Check sheet for the modelled part. Datum: model origin and axes. Units: mm. A direction names the side the tool comes from. Round coordinates to 2 decimals unless told otherwise and drop trailing zeros. Loops run counter-clockwise (first coordinate to the right, second up) from the corner with the lowest first, then second, coordinate; pieces in that order, holes last. Notation, with made-up numbers: (9.5, 48.5) - (24.5, 48.5) arc R27 cw to (24.5, 64.5) - close; hole circle Ø10 at (58.5, -6.5). An arc over 180 degrees is marked (long way). Answer in a Markdown table with one row per item. Add a question column.
(1) Thickness scan on line 1 along Y through (x, z) = (1.75, 3.5); line 2 along Z through (x, y) = (5.5, -12); line 3 along Y through (x, z) = (5.25, -3). Record the ranges inside material, lowest first.
(2) Cross-section at C-C on y = -16.5. Enter the section's corners in (x, z), then the cut area to 3 significant figures.
(3) Mould release check, pull along Z, two halves, no side actions. Record for faces 1 (the flat face through (-4.02, 0, 4)), 2 (the flat face through (0.532, -2.776, 3.095)), 3 (the flat face through (5.259, -26.016, -31.007)): +Z half, -Z half, draft (parallel to the pull), parting line (faces both ways), or undercut.
(4) Gauge pin test, flat ends, axial feed: pin 1 (1.6 mm diameter, centred on x = 5.5, z = 4.5, fed in from +Y); pin 2 (0.6 mm diameter, centred on y = -3.5, z = 4, fed in from +X); pin 3 (1.5 mm diameter, centred on y = -24.5, z = -32, fed in from +X). Record the tip position at first contact, or that the pin passes through.
(5) Cross-section at B-B on z = -11. Enter the section's corners in (x, y).
(6) Access from +Z, -Z, +X, -X, +Y, -Y to the whole of each face (thin tool, end or side, straight path). Record for faces 4 (the cylindrical face through (-0.69, -25.64, -30.54)), 5 (the flat face through (0.5, -20.6, -33.8)), 6 (the flat face through (-0.08, -22.91, -26.23)), 7 (the flat face through (0, 0, 0)).
from build123d import *

# Parameters (mm, degrees)
SKETCH1_W                      = 12.04
SKETCH1_H                      = 7.58
SKETCH1_W_2                    = 8.04
SKETCH1_H_2                    = 3.58
BOSS_EXTRUDE1_DEPTH            = 8
SKETCH1_2_W                    = 12.04
SKETCH1_2_H                    = 7.58
SKETCH1_2_W_2                  = 8.04
SKETCH1_2_H_2                  = 3.58
BOSS_EXTRUDE2_DEPTH            = 2
EXTRUDE_THIN1_DEPTH            = 12.04
SKETCH5_W                      = 12.04
SKETCH5_H                      = 7.58
SKETCH5_W_2                    = 8.04
SKETCH5_H_2                    = 3.58
BOSS_EXTRUDE4_DEPTH            = 8
SKETCH5_4_W                    = 12.04
SKETCH5_4_H                    = 7.58
BOSS_EXTRUDE5_DEPTH            = 2
CHAMFER1_SIZE                  = 1.5
CHAMFER2_START                 = -7
CHAMFER2_DEPTH                 = 14
CUT_EXTRUDE1_REACH             = 50.973
CUT_EXTRUDE1_DIRECTION_2_DEPTH = 49.973440368
CUT_EXTRUDE2_DEPTH             = 48.541116576
CUT_EXTRUDE2_DEPTH_BACK        = 48.541116576
SKETCH8_W                      = 2
SKETCH8_H                      = 1.58
CUT_EXTRUDE3_DEPTH             = 6.5
SKETCH9_W                      = 4
SKETCH9_H                      = 1.58
CUT_EXTRUDE4_DEPTH             = 6.5
CHAMFER3_SIZE                  = 0.5
SKETCH10_W                     = 0.414634146
SKETCH10_H                     = 2
SKETCH10_W_2                   = 0.414634147
BOSS_EXTRUDE6_DEPTH            = 0.3


with BuildPart() as part:
    # Sketch1 → Boss-Extrude1 (new body)
    with BuildSketch(Plane.XY):
        Rectangle(SKETCH1_W, SKETCH1_H)
        Rectangle(SKETCH1_W_2, SKETCH1_H_2, mode=Mode.SUBTRACT)
    extrude(amount=BOSS_EXTRUDE1_DEPTH)

    # Sketch1<2> → Boss-Extrude2 (add)
    # profile 1 of 2: a face of its own
    with BuildSketch(Plane.XY):
        Rectangle(SKETCH1_2_W, SKETCH1_2_H)
        Rectangle(SKETCH1_2_W_2, SKETCH1_2_H_2, mode=Mode.SUBTRACT)
    # profile 2 of 2: a face of its own
    with BuildSketch(Plane.XY):
        Rectangle(SKETCH1_2_W_2, SKETCH1_2_H_2)
    extrude(amount=-BOSS_EXTRUDE2_DEPTH)

    # Sketch3 → Extrude-Thin1 (add)
    with BuildSketch(Plane(origin=(6.02, 9.81, 0), x_dir=(0, -1, 0), z_dir=(1, 0, 0))):
        with BuildLine():
            Line((6.02, 2.744137986), (6.52, 2.744137986))
            ThreePointArc((6.52, 2.744137986), (10.07949931, 2.557592532), (13.6, 2))
            Line((13.6, 2), (21.425180806, 0.336706473))
            ThreePointArc((21.425180806, 0.336706473), (22.120268588, 0.441550315), (22.574623539, 0.977927827))
            ThreePointArc((22.574623539, 0.977927827), (26.849152106, 14.317688881), (30.219561316, 27.914054616))
            Line((30.219561316, 27.914054616), (30.401286915, 28.769006338))
            Line((30.401286915, 28.769006338), (32.357582116, 28.353182957))
            Line((32.357582116, 28.353182957), (32.175856518, 27.498231234))
            ThreePointArc((32.175856518, 27.498231234), (28.773161162, 13.771621897), (24.457685624, 0.304075332))
            ThreePointArc((24.457685624, 0.304075332), (23.094620772, -1.305057203), (21.009357424, -1.619588728))
            Line((21.009357424, -1.619588728), (13.184176618, 0.043704799))
            ThreePointArc((13.184176618, 0.043704799), (9.870442383, 0.568548741), (6.52, 0.744137986))
            Line((6.52, 0.744137986), (6.02, 0.744137986))
            Line((6.02, 0.744137986), (6.02, 2.744137986))
        make_face()
    extrude(amount=-EXTRUDE_THIN1_DEPTH)



with BuildPart() as body_2:
    # Sketch5 → Boss-Extrude4 (new body)
    with BuildSketch(Plane(origin=(0, 484.189145571, -136.063399466), x_dir=(1, 0, 0), z_dir=(0, -0.20791169081775487, -0.9781476007338067))):
        with Locations((0, 517.847527624)):
            Rectangle(SKETCH5_W, SKETCH5_H)
        with Locations((0, 517.847527624)):
            Rectangle(SKETCH5_W_2, SKETCH5_H_2, mode=Mode.SUBTRACT)
    extrude(amount=BOSS_EXTRUDE4_DEPTH)


with BuildPart() as part_1:
    add(part.part)

    add(body_2.part)  # Boss-Extrude5 merges body 2
    # Sketch5<4> → Boss-Extrude5 (add)
    with BuildSketch(Plane(origin=(0, 484.189145571, -136.063399466), x_dir=(1, 0, 0), z_dir=(0, -0.20791169081775487, -0.9781476007338067))):
        with Locations((0, 517.847527624)):
            Rectangle(SKETCH5_4_W, SKETCH5_4_H)
    extrude(amount=-BOSS_EXTRUDE5_DEPTH)

    # Chamfer1
    chamfer1_edges = [part_1.edges().sort_by_distance(p)[0] for p in [
        (6.02, -26.673085599, -30.543301906),
        (-6.02, -26.673085599, -30.543301906),
        (6.02, 3.79, 2.627931007),
        (6.02, -3.79, 4.022340595),
        (-6.02, -3.79, 4.022340595),
        (-6.02, 3.79, 2.627931007),
        (6.02, -19.258726786, -32.119272522),
        (-6.02, -19.258726786, -32.119272522),
    ]]
    chamfer(chamfer1_edges, length=CHAMFER1_SIZE)

    # Chamfer2: read off the stored shape, not the designer's step
    # Chamfer2 outline → Chamfer2 (cut)
    with BuildSketch(Plane.YZ.offset(CHAMFER2_START)):
        with BuildLine():
            Line((3.79, -2.744137986), (3.79, -0.709020541))
            Line((3.79, -0.709020541), (1.696404781, -2.706829325))
            ThreePointArc((1.696404781, -2.706829325), (2.492984056, -2.734809543), (3.29, -2.744137986))
            Line((3.29, -2.744137986), (3.79, -2.744137986))
        make_face()
        Polygon((-25.633527145, -25.652563902), (-26.049350527, -27.608859104), (-23.677231944, -26.068387284), align=None)
        with BuildLine():
            ThreePointArc((-20.172493797, -26.813342374), (-20.172815684, -26.814817596), (-20.173137561, -26.81629282))
            Line((-20.173137561, -26.81629282), (-18.634991713, -29.18482972))
            Line((-18.634991713, -29.18482972), (-18.219168332, -27.228534519))
            Line((-18.219168332, -27.228534519), (-20.172493797, -26.813342374))
        make_face()
    extrude(amount=CHAMFER2_DEPTH, mode=Mode.SUBTRACT)

    # Cut-Extrude1: up to this face of the body (flat: up to its plane)
    cut_extrude1_end = Plane(part_1.part.faces().sort_by_distance((0, -3.79, 4.022340595))[0])
    # Sketch6 → Cut-Extrude1 (cut, up to the picked face)
    with BuildSketch(Plane(origin=(0, 3.79, 0), x_dir=(1, 0, 0), z_dir=(0, 1, 0)), mode=Mode.PRIVATE) as cut_extrude1_sk1:
        with BuildLine():
            Line((1.05, -3.393782217), (0, -2.787564435))
            ThreePointArc((0, -2.787564435), (-0.7, -2.787564435), (-1.05, -3.393782217))
            Line((-1.05, -3.393782217), (-1.05, -4.606217783))
            ThreePointArc((-1.05, -4.606217783), (-0.7, -5.212435565), (0, -5.212435565))
            Line((0, -5.212435565), (1.05, -4.606217783))
            ThreePointArc((1.05, -4.606217783), (1.4, -4), (1.05, -3.393782217))
        make_face()
    cut_extrude1_tool1 = split(extrude(cut_extrude1_sk1.sketch, amount=-CUT_EXTRUDE1_REACH, mode=Mode.PRIVATE), bisect_by=cut_extrude1_end, keep=Keep.BOTH, mode=Mode.PRIVATE)
    add(cut_extrude1_tool1.solids().sort_by(Axis((0, 3.79, 4), (0, -1, 0)))[0], mode=Mode.SUBTRACT)

    # Sketch6 → Cut-Extrude1 direction 2 (cut)
    with BuildSketch(Plane(origin=(0, 3.79, 0), x_dir=(1, 0, 0), z_dir=(0, 1, 0))):
        with BuildLine():
            Line((1.05, -3.393782217), (0, -2.787564435))
            ThreePointArc((0, -2.787564435), (-0.7, -2.787564435), (-1.05, -3.393782217))
            Line((-1.05, -3.393782217), (-1.05, -4.606217783))
            ThreePointArc((-1.05, -4.606217783), (-0.7, -5.212435565), (0, -5.212435565))
            Line((0, -5.212435565), (1.05, -4.606217783))
            ThreePointArc((1.05, -4.606217783), (1.4, -4), (1.05, -3.393782217))
        make_face()
    extrude(amount=CUT_EXTRUDE1_DIRECTION_2_DEPTH, mode=Mode.SUBTRACT)

    # Sketch7 → Cut-Extrude2 (cut, two sides: drawn at the far end of the back side and taken through both)
    with BuildSketch(Plane(origin=(0, -19.308540852, 4.104157054), x_dir=(1, 0, 0), z_dir=(0, -0.9781476007338067, 0.2079116908177549)).offset(-CUT_EXTRUDE2_DEPTH_BACK)):
        with BuildLine():
            Line((1.05, -35.815286021), (0, -35.209068239))
            ThreePointArc((0, -35.209068239), (-0.7, -35.209068239), (-1.05, -35.815286021))
            Line((-1.05, -35.815286021), (-1.05, -37.027721587))
            ThreePointArc((-1.05, -37.027721587), (-0.7, -37.633939369), (0, -37.633939369))
            Line((0, -37.633939369), (1.05, -37.027721587))
            ThreePointArc((1.05, -37.027721587), (1.4, -36.421503804), (1.05, -35.815286021))
        make_face()
    extrude(amount=CUT_EXTRUDE2_DEPTH + CUT_EXTRUDE2_DEPTH_BACK, mode=Mode.SUBTRACT)

    # Sketch8 → Cut-Extrude3 (cut)
    with BuildSketch(Plane.XY.offset(8)):
        with Locations((5.02, 0)):
            Rectangle(SKETCH8_W, SKETCH8_H)
    extrude(amount=-CUT_EXTRUDE3_DEPTH, mode=Mode.SUBTRACT)

    # Sketch9 → Cut-Extrude4 (cut)
    with BuildSketch(Plane(origin=(0, -8.404103201, -39.538196964), x_dir=(-1, 0, 0), z_dir=(0, -0.20791169081775673, -0.9781476007338064))):
        with Locations((-6.02, -15.949905141)):
            Rectangle(SKETCH9_W, SKETCH9_H)
    extrude(amount=-CUT_EXTRUDE4_DEPTH, mode=Mode.SUBTRACT)

    # Chamfer3
    chamfer3_edges = [part_1.edges().sort_by_distance(p)[0] for p in [
        (4.02, -0.79, 4.75),
        (4.02, 0.79, 4.75),
        (4.02, 0, 1.5),
        (4.02, -24.102488256, -32.87879528),
        (4.02, -22.654038656, -29.864065813),
        (4.02, -22.557015047, -33.207295751),
    ]]
    chamfer(chamfer3_edges, length=CHAMFER3_SIZE)

    # Sketch10 → Boss-Extrude6 (add)
    with BuildSketch(Plane(origin=(6.02, 0, 0), x_dir=(0, 0, -1), z_dir=(1, 0, 0))):
        with Locations((0.149293265, -0.21)):
            Rectangle(SKETCH10_W, SKETCH10_H)
        with Locations((1.027342045, -0.21)):
            Rectangle(SKETCH10_W_2, SKETCH10_H)
    extrude(amount=BOSS_EXTRUDE6_DEPTH)


solid = part_1.part
Answers:
| question | item | result |
|---|---|---|
| 1 | line 1 | y = -3.79 to -1.79, 1.79 to 3.79 |
| 1 | line 2 | z = -0.33 to 1.68 |
| 1 | line 3 | y = -15.59 to -13.48 |
| 2 | outline | (-6.02, -12.45) - (6.02, -12.45) - (6.02, -5.71) - (-6.02, -5.71) - close |
| 2 | area | 81.2 mm^2 |
| 3 | face 1 | draft |
| 3 | face 2 | undercut |
| 3 | face 3 | +Z half |
| 4 | pin 1 | stops at y = 3.61 |
| 4 | pin 2 | stops at x = 5.11 |
| 4 | pin 3 | stops at x = 6.02 |
| 5 | outline | (-6.02, -18.16) - (6.02, -18.16) - (6.02, -16.07) - (-6.02, -16.07) - close |
| 6 | face 4 | -Y |
| 6 | face 5 | +Y |
| 6 | face 6 | +Z, +X, -X |
| 6 | face 7 | +Z |
